Part model, mm, in its own coordinate system. Face numbers are marked on the shaded views. Give positions to 0.01 mm unless a question says otherwise; leave off trailing zeros. Write each loop counter-clockwise with the first axis right and the second up, starting at its lowest first coordinate (ties: lowest second). Pieces come first, ordered by that corner, then holes. Notation, with made-up numbers: M 46.5,37 L 81.5,37 A15 cw 81.5,58 Z; hole C 79.5,-27.75 d8. An arc over 180 degrees is marked long. Use CSV: the item, a comma, the result in double quotes. Start each with the question number.
Item 1: Pin check, flat tips, straight feed: pin 1 (3.5 mm diameter, centred on x = -9, y = 83.08, fed in from +Z); pin 2 (2.5 mm diameter, centred on x = -17.5, y = 76.5, fed in from -Z). Stop position of each tip, or through.
Item 2: Cut at B-B (y = 104). List the corners of the cut face in (x, z).
Item 3: Cut at A-A (y = 89). List the corners of the cut face in (x, z), then the cut area to 3 significant figures.
Item 4: Mould opens along Y. For the marked faces 1, 2 and 3 say: released by +Y, released by -Y, zero draft, split by the parting line, or undercut.
Item 5: Drill centre lines: line 1 (X direction, y = 76.5, z = -2); line 2 (Y direction, x = 2.5, z = -2.25); line 3 (Z direction, x = 15, y = 7.25). Where is each one in solid material? Low to high. Write a range as [from, to].
from build123d import *

# Parameters (mm, degrees)
SKIZZE1_W                                            = 45
SKIZZE1_H                                            = 140
AUFSATZ_LINEAR_AUSTRAGEN1_DEPTH                      = 5
STIRNSENKUNG_F_R_M4_ZYLINDERSCHRAUBE_MIT_D           = 4.5
STIRNSENKUNG_F_R_M4_ZYLINDERSCHRAUBE_MIT_CBORE_D     = 8
STIRNSENKUNG_F_R_M4_ZYLINDERSCHRAUBE_MIT_CBORE_DEPTH = 4.4
M5_GEWINDEBOHRUNG1_D                                 = 4.2
LINEARES_MUSTER1_COUNT                               = 2
LINEARES_MUSTER1_PITCH                               = 20
M5_GEWINDEBOHRUNG2_D                                 = 4.2
M5_GEWINDEBOHRUNG2_DEPTH                             = 14
M5_GEWINDEBOHRUNG2_TIP                               = 1.2618073
F_4_0_4_DURCHMESSER_BOHRUNG1_D                       = 4
F_4_0_4_DURCHMESSER_BOHRUNG1_DEPTH                   = 14
F_4_0_4_DURCHMESSER_BOHRUNG1_TIP                     = 1.201721238
F_3_0_3_DURCHMESSER_BOHRUNG1_D                       = 3
F_3_0_3_DURCHMESSER_BOHRUNG1_DEPTH                   = 8
F_20_0_20_DURCHMESSER_BOHRUNG1_D                     = 20


with BuildPart() as part:
    # Skizze1 → Aufsatz-Linear austragen1 (new, symmetric)
    with BuildSketch(Plane.XY):
        with Locations((0, 70)):
            Rectangle(SKIZZE1_W, SKIZZE1_H)
    extrude(amount=AUFSATZ_LINEAR_AUSTRAGEN1_DEPTH, both=True)

    # Stirnsenkung für M4 Zylinderschraube mit Innensechskant1 (through all)
    with Locations(Plane.XY.offset(5)):
        with Locations((-9, 83.08)):
            stirnsenkung_f_r_m4_zylinderschraube_mit = CounterBoreHole(STIRNSENKUNG_F_R_M4_ZYLINDERSCHRAUBE_MIT_D / 2, STIRNSENKUNG_F_R_M4_ZYLINDERSCHRAUBE_MIT_CBORE_D / 2, STIRNSENKUNG_F_R_M4_ZYLINDERSCHRAUBE_MIT_CBORE_DEPTH)

    # M5 Gewindebohrung1 (through all)
    with Locations(Plane.XY.offset(5)):
        with Locations((15, 119), (-15, 89), (-15, 119), (15, 89)):
            Hole(M5_GEWINDEBOHRUNG1_D / 2)

    # Lineares Muster1: Stirnsenkung für M4 Zylinderschraube mit Innensechskant1 ×2
    with Locations(*[(0, -i * LINEARES_MUSTER1_PITCH, 0) for i in range(1, LINEARES_MUSTER1_COUNT)]):
        add(stirnsenkung_f_r_m4_zylinderschraube_mit, mode=Mode.SUBTRACT)

    # M5 Gewindebohrung2
    with Locations(Plane(origin=(0, 0, 0), x_dir=(-1, 0, 0), z_dir=(0, -1, 0))):
        with Locations((0, 0)):
            Hole(M5_GEWINDEBOHRUNG2_D / 2, depth=M5_GEWINDEBOHRUNG2_DEPTH)
            with Locations((0, 0, -(M5_GEWINDEBOHRUNG2_DEPTH + M5_GEWINDEBOHRUNG2_TIP / 2))):  # 118° drill point
                Cone(0, M5_GEWINDEBOHRUNG2_D / 2, M5_GEWINDEBOHRUNG2_TIP, mode=Mode.SUBTRACT)

    # Ø4.0 (4) Durchmesser Bohrung1
    with Locations(Plane(origin=(0, 0, 0), x_dir=(-1, 0, 0), z_dir=(0, -1, 0))):
        with Locations((15, 0), (-15, 0)):
            Hole(F_4_0_4_DURCHMESSER_BOHRUNG1_D / 2, depth=F_4_0_4_DURCHMESSER_BOHRUNG1_DEPTH)
            with Locations((0, 0, -(F_4_0_4_DURCHMESSER_BOHRUNG1_DEPTH + F_4_0_4_DURCHMESSER_BOHRUNG1_TIP / 2))):  # 118° drill point
                Cone(0, F_4_0_4_DURCHMESSER_BOHRUNG1_D / 2, F_4_0_4_DURCHMESSER_BOHRUNG1_TIP, mode=Mode.SUBTRACT)

    # Ø3.0 (3) Durchmesser Bohrung1
    with Locations(Plane(origin=(0, 0, -5), x_dir=(-1, 0, 0), z_dir=(0, 0, -1))):
        with Locations((17.5, 76.5), (-2.5, 76.5)):
            Hole(F_3_0_3_DURCHMESSER_BOHRUNG1_D / 2, depth=F_3_0_3_DURCHMESSER_BOHRUNG1_DEPTH)

    # Ø20.0 (20) Durchmesser Bohrung1 (through all)
    with Locations(Plane(origin=(0, 0, -5), x_dir=(-1, 0, 0), z_dir=(0, 0, -1))):
        with Locations((0, 104)):
            Hole(F_20_0_20_DURCHMESSER_BOHRUNG1_D / 2)


solid = part.part
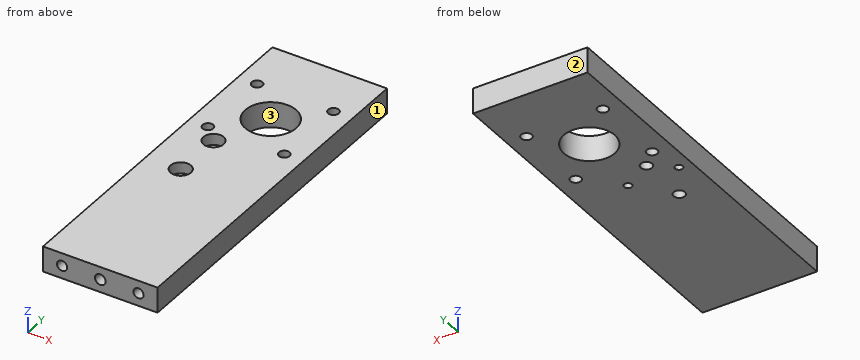
Worked answers:
1,pin 1,"passes through"
1,pin 2,"stops at z = 3"
2,outline,"M -22.5,-5 L -10,-5 L -10,5 L -22.5,5 Z; M 10,-5 L 22.5,-5 L 22.5,5 L 10,5 Z"
3,outline,"M -22.5,-5 L -17.1,-5 L -17.1,5 L -22.5,5 Z; M -12.9,-5 L 12.9,-5 L 12.9,5 L -12.9,5 Z; M 17.1,-5 L 22.5,-5 L 22.5,5 L 17.1,5 Z"
3,area,"366 mm^2"
4,face 1,"zero draft"
4,face 2,"released by +Y"
4,face 3,"undercut"
5,line 1,"x = [-22.5, -19], [-16, 1], [4, 22.5]"
5,line 2,"y = [0, 75], [78, 94.32], [113.68, 140]"
5,line 3,"z = [-5, -2], [2, 5]"
